Here's how the part is built. I have some questions about the finished solid (model axes, mm). Face numbers are marked on the shaded views. A direction names the side the tool comes from. Coordinates: 2 decimals unless noted, no trailing zeros. Write each loop counter-clockwise with the first axis right and the second up, starting at its lowest first coordinate (ties: lowest second). Pieces come first, ordered by that corner, then holes.
from build123d import *

# Parameters (mm, degrees)
SKETCH_1_R          = 15
SKETCH_1_R_2        = 1.86
EXTRUDE_1_DEPTH     = 3.7
SKETCH_2_R          = 15
EXTRUDE_2_DEPTH     = 1.6
SKETCH_3_R          = 8.5
EXTRUDE_3_DEPTH     = 0.4
SKETCH_4_R          = 7.5
EXTRUDE_4_DEPTH     = 6.5
SKETCH_5_R          = 1.25
SKETCH_5_R_2        = 2.5
CUT_EXTRUDE_1_DEPTH = 7
CHAMFER_1_SIZE      = 0.2
SKETCH_7_R          = 2.5
CUT_EXTRUDE_4_DEPTH = 23.338307904
SKETCH_8_R          = 6
CUT_EXTRUDE_5_DEPTH = 2
CHAMFER_2_SIZE      = 0.5


with BuildPart() as part:
    # 草图1 → 凸台-拉伸1 (new body)
    with BuildSketch(Plane(origin=(0, 0, 0), x_dir=(1, 0, 0), z_dir=(0, 1, 0))):
        with Locations(Location((0, 0, 0), (0, 0, 270))):
            Circle(SKETCH_1_R)
        with Locations(Location((0, 11.525, 0), (0, 0, 270))):
            Circle(SKETCH_1_R_2, mode=Mode.SUBTRACT)
        with Locations(Location((9.980942779, 5.7625, 0), (0, 0, 270))):
            Circle(SKETCH_1_R_2, mode=Mode.SUBTRACT)
        with Locations(Location((9.980942779, -5.7625, 0), (0, 0, 270))):
            Circle(SKETCH_1_R_2, mode=Mode.SUBTRACT)
        with Locations(Location((0, -11.525, 0), (0, 0, 270))):
            Circle(SKETCH_1_R_2, mode=Mode.SUBTRACT)
        with Locations(Location((-9.980942779, -5.7625, 0), (0, 0, 270))):
            Circle(SKETCH_1_R_2, mode=Mode.SUBTRACT)
        with Locations(Location((-9.980942779, 5.7625, 0), (0, 0, 270))):
            Circle(SKETCH_1_R_2, mode=Mode.SUBTRACT)
    extrude(amount=EXTRUDE_1_DEPTH)

    # 草图2 → 凸台-拉伸2 (add)
    with BuildSketch(Plane(origin=(0, 3.7, 0), x_dir=(1, 0, 0), z_dir=(0, 1, 0))):
        with Locations(Location((0, 0, 0), (0, 0, 270))):
            Circle(SKETCH_2_R)
    extrude(amount=EXTRUDE_2_DEPTH)

    # 草图3 → 凸台-拉伸3 (add)
    with BuildSketch(Plane(origin=(0, 5.3, 0), x_dir=(1, 0, 0), z_dir=(0, 1, 0))):
        with Locations(Location((0, 0, 0), (0, 0, 270))):
            Circle(SKETCH_3_R)
    extrude(amount=EXTRUDE_3_DEPTH)

    # 草图4 → 凸台-拉伸4 (add)
    with BuildSketch(Plane(origin=(0, 5.7, 0), x_dir=(1, 0, 0), z_dir=(0, 1, 0))):
        with Locations(Location((0, 0, 0), (0, 0, 90))):
            Circle(SKETCH_4_R)
    extrude(amount=EXTRUDE_4_DEPTH)

    # 草图5 → 切除-拉伸1 (cut)
    with BuildSketch(Plane(origin=(0, 12.2, 0), x_dir=(1, 0, 0), z_dir=(0, 1, 0))):
        with Locations(Location((0, 5, 0), (0, 0, 270))):
            Circle(SKETCH_5_R)
        with Locations(Location((5, 0, 0), (0, 0, 270))):
            Circle(SKETCH_5_R)
        with Locations(Location((0, -5, 0), (0, 0, 270))):
            Circle(SKETCH_5_R)
        with Locations(Location((-5, 0, 0), (0, 0, 270))):
            Circle(SKETCH_5_R)
        with Locations(Location((0, 0, 0), (0, 0, 270))):
            Circle(SKETCH_5_R_2)
    extrude(amount=-CUT_EXTRUDE_1_DEPTH, mode=Mode.SUBTRACT)

    # 倒角1
    chamfer_1_edges = [part.edges().sort_by_distance(p)[0] for p in [
        (9.980942779, 0, 3.9025),
        (0, 0, 9.665),
        (0, 0, -15),
        (-9.980942779, 0, 3.9025),
        (-9.980942779, 0, -7.6225),
        (0, 5.3, -15),
        (0, 12.2, 7.5),
        (0, 0, -13.385),
        (0, 12.2, -2.5),
        (9.980942779, 0, -7.6225),
    ]]
    chamfer(chamfer_1_edges, length=CHAMFER_1_SIZE)

    # 草图7 → 切除-拉伸4 (cut, through all)
    with BuildSketch(Plane(origin=(0, 5.2, 0), x_dir=(1, 0, 0), z_dir=(0, 1, 0))):
        with Locations(Location((0, 0, 0), (0, 0, 270))):
            Circle(SKETCH_7_R)
    extrude(amount=-CUT_EXTRUDE_4_DEPTH, mode=Mode.SUBTRACT)

    # 草图8 → 切除-拉伸5 (cut)
    with BuildSketch(Plane(origin=(0, 0, 0), x_dir=(-1, 0, 0), z_dir=(0, -1, 0))):
        with Locations(Location((0, 0, 0), (0, 0, 90))):
            Circle(SKETCH_8_R)
    extrude(amount=-CUT_EXTRUDE_5_DEPTH, mode=Mode.SUBTRACT)

    # 倒角2
    chamfer_2_edges = [part.edges().sort_by_distance(p)[0] for p in [
        (0, 0, 6),
        (0, 2, 6),
        (0, 2, -2.5),
    ]]
    chamfer(chamfer_2_edges, length=CHAMFER_2_SIZE)


solid = part.part
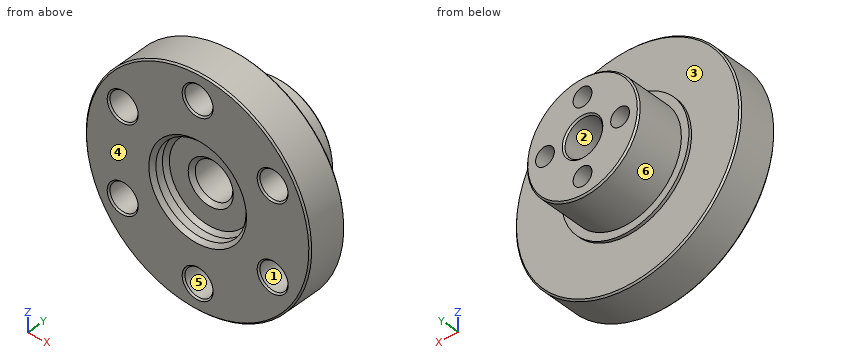
1. I want a section at A-A (y = 9.75). List the corners of the cut face in (x, z) for me.
2. Thinking about a two-plate mould opening in X: for the marked faces 4, 5 and 6, which applies, pulls with the +X half, pulls with the -X half, needs draft (parallel to the pull), parting line crosses it, or undercut?
3. On a 3-axis mill with a long thin cutter (end or side, diameter ignored), from which of +Z, -Z, +X, -X, +Y, -Y can I reach the whole of each face in a straight line? I mean the marked faces 1, 2 and 3. Say none if no direction works.
4. If I drill on line 1 (X direction, y = 9, z = 0); line 2 (X direction, y = 10.5, z = -0.5); line 3 (Y direction, x = 1.25, z = -10.5), over which ranges is the centre line in solid material (lowest first)?
5. For pin 1 Ø6 at (x, y) = (-12, 7.5) entering from +Z; pin 2 Ø1 at (y, z) = (2.5, 1.5) entering from +X; pin 3 Ø4 at (y, z) = (1.5, 4.5) entering from -X; pin 4 Ø2 at (x, z) = (-0.5, -4.5) entering from +Y, each with a flat end and sliding along its axis, tell me the tip position at first contact or that it passes through.
6. I want a section at B-B (y = 1). List the corners of the cut face in (x, z) for me (1 decimal), then the cut area to 3 significant figures.
Response values:
1. outline: circle Ø15 at (0, 0); hole circle Ø2.5 at (-5, 0); hole circle Ø5 at (0, 0); hole circle Ø2.5 at (0, -5); hole circle Ø2.5 at (0, 5); hole circle Ø2.5 at (5, 0)
2. face 4: needs draft
2. face 5: undercut
2. face 6: parting line crosses it
3. face 1: -Y
3. face 2: +Y, -Y
3. face 3: +Y
4. line 1: x = -7.5 to -6.25, -3.75 to -2.5, 2.5 to 3.75, 6.25 to 7.5
4. line 2: x = -7.48 to -6.15, -3.85 to -2.45, 2.45 to 3.85, 6.15 to 7.48
4. line 3: y = 3.7 to 5.3
5. pin 1: stops at z = 11
5. pin 2: stops at x = 14.97
5. pin 3: stops at x = -14.79
5. pin 4: stops at y = 12.2
6. outline: circle Ø30 at (0, 0); hole circle Ø3.7 at (-10, -5.8); hole circle Ø3.7 at (-10, 5.8); hole circle Ø12 at (0, 0); hole circle Ø3.7 at (0, -11.5); hole circle Ø3.7 at (0, 11.5); hole circle Ø3.7 at (10, -5.8); hole circle Ø3.7 at (10, 5.8)
6. area: 529 mm2
